For this review, take the finished solid that the model builds, in its own axes (mm). Coordinates: 2 decimals unless noted, no trailing zeros. Loops run counter-clockwise (first coordinate to the right, second up) from the corner with the lowest first, then second, coordinate; pieces in that order, holes last. Notation, with made-up numbers: (-36.75, 33) - (11.25, 33) arc R29 cw to (11.25, 61) - close; hole circle Ø5 at (-18, -22). An arc over 180 degrees is marked (long way). One line per item, written item: value. Start each with the question number.
1. Take a section at B-B, the plane x = 0. State the section outline as (y, z) points.
2. To check wall thickness, follow line 1 (Y direction, x = 11.5, z = 11.75); line 2 (Y direction, x = -8, z = 6); line 3 (X direction, y = 11, z = 26.5). State the ranges of each line that lie inside material, in increasing order. Write a range as from..to.
3. The part is to be moulded in two halves that separate along X. For faces 1 (the face through (-8, 8, 29)), 2 (the face through (-12.838, 4.176, 14.297)), say which applies: released by +X, released by -X, zero draft, split by the parting line, or undercut.
4. Insertion check: pin 1 (2 mm diameter, centred on y = -12, z = 19, fed in from -X); pin 2 (3 mm diameter, centred on y = -10, z = 11, fed in from -X); pin 3 (3 mm diameter, centred on x = -3.5, z = 8, fed in from +Y). Each pin has a flat end and moves straight along its axis. Give the tip position at first contact, or say it passes through.
5. Take a section at A-A, the plane y = 0. State the section outline as (x, z) points, and give its area (3 significant figures).
Autodesk Inventor part; units mm, degrees
ref_plane "YZ Plane" through (0, 0, 0) normal (1, 0, 0) x (0, 1, 0)
ref_plane "XZ Plane" through (0, 0, 0) normal (0, 1, 0) x (-1, 0, 0)
ref_plane "XY Plane" through (0, 0, 0) normal (0, 0, 1) x (1, 0, 0)
sketch "Sketch1" plane through (0, 0, 0) normal (0, 0, 1) x (1, 0, 0)
  arc A0 (-10.8205, 1.9793) -> (-10.8147, -2.0103) centre (0, 0) ccw
  line L0 (-10.8147, -2.0103) -> (-13.2812, -2.8117)
  line L1 (-12.3877, -5.5615) -> (-13.2812, -2.8117)
  line L2 (-13.2812, -2.8117) -> (-12.3877, -5.5615)
  line L3 (-12.3877, -5.5615) -> (-9.9173, -4.7588)
  line L4 (-12.3974, 5.5317) -> (-13.2908, 2.782)
  line L5 (-13.2908, 2.782) -> (-10.8205, 1.9793)
  line L6 (-9.931, 4.7303) -> (-12.3974, 5.5317)
  arc A1 (-7.5905, 7.9614) -> (-9.931, 4.7303) centre (0, 0) ccw
  line L7 (-6.7782, 11.7623) -> (-9.1173, 10.0628)
  line L8 (-9.1173, 10.0628) -> (-7.5905, 7.9614)
  line L9 (-5.2539, 9.6642) -> (-6.7782, 11.7623)
  arc A2 (-1.4613, 10.9025) -> (-5.2539, 9.6642) centre (0, 0) ccw
  line L10 (1.43, 13.5) -> (-1.4613, 13.5)
  line L11 (-1.4613, 13.5) -> (-1.4613, 10.9025)
  line L12 (1.43, 10.9067) -> (1.43, 13.5)
  arc A3 (5.2261, 9.6792) -> (1.43, 10.9067) centre (0, 0) ccw
  line L13 (9.092, 10.0812) -> (6.7529, 11.7806)
  line L14 (6.7529, 11.7806) -> (5.2261, 9.6792)
  line L15 (7.5677, 7.9831) -> (9.092, 10.0812)
  arc A4 (9.9173, 4.7588) -> (7.5677, 7.9831) centre (0, 0) ccw
  line L16 (13.2812, 2.8117) -> (12.3877, 5.5615)
  line L17 (12.3877, 5.5615) -> (9.9173, 4.7588)
  line L18 (10.8147, 2.0103) -> (13.2812, 2.8117)
  arc A5 (10.8205, -1.9793) -> (10.8147, 2.0103) centre (0, 0) ccw
  line L19 (12.3974, -5.5317) -> (13.2908, -2.782)
  line L20 (13.2908, -2.782) -> (10.8205, -1.9793)
  line L21 (9.931, -4.7303) -> (12.3974, -5.5317)
  arc A6 (7.5905, -7.9614) -> (9.931, -4.7303) centre (0, 0) ccw
  line L22 (6.7782, -11.7623) -> (9.1173, -10.0628)
  line L23 (9.1173, -10.0628) -> (7.5905, -7.9614)
  line L24 (5.2539, -9.6642) -> (6.7782, -11.7623)
  arc A7 (1.4613, -10.9025) -> (5.2539, -9.6642) centre (0, 0) ccw
  line L25 (-1.43, -13.5) -> (1.4613, -13.5)
  line L26 (1.4613, -13.5) -> (1.4613, -10.9025)
  line L27 (-1.43, -10.9067) -> (-1.43, -13.5)
  arc A8 (-5.2261, -9.6792) -> (-1.43, -10.9067) centre (0, 0) ccw
  line L28 (-9.092, -10.0812) -> (-6.7529, -11.7806)
  line L29 (-6.7529, -11.7806) -> (-5.2261, -9.6792)
  line L30 (-7.5677, -7.9831) -> (-9.092, -10.0812)
  arc A9 (-9.9173, -4.7588) -> (-7.5677, -7.9831) centre (0, 0) ccw
  circle A10 centre (0, 0) radius 17
  circle A11 centre (0, 0) radius 8.5
  point P0 (-10.8205, 1.9793)
  point P1 (-7.5905, 7.9614)
  point P2 (5.2261, 9.6792)
  point P3 (9.9173, 4.7588)
  point P4 (10.8205, -1.9793)
  point P5 (7.5905, -7.9614)
  point P6 (1.4613, -10.9025)
  point P7 (-5.2261, -9.6792)
  point P8 (-9.9173, -4.7588)
  dimension "d2" = 360
  dimension "d3" = 34
  dimension "d6" = 11
  dimension "d7" = 17
  dimension "d8" = 2.5933
  dimension "d9" = 2.8912
extrude "Extrusion1" add sketch "Sketch1" along normal blind 29 contours A10
properties part number "opona"
Solutions:
1. outline: (-17, 0) - (-13.5, 0) - (-13.5, 29) - (-17, 29) - close; (13.5, 0) - (17, 0) - (17, 29) - (13.5, 29) - close
2. line 1: -12.52..-5.24, -2.2..2.23, 5.27..12.52
2. line 2: -15..-10.87, -8.58..-7.55, 7.55..8.53, 10.87..15
2. line 3: -12.96..-7.83, -6.22..-1.46, 1.43..6.19, 7.83..12.96
3. face 1: zero draft
3. face 2: undercut
4. pin 1: x = -12.96
4. pin 2: x = -14.72
4. pin 3: y = 16.88
5. outline: (-17, 0) - (-11, 0) - (-11, 29) - (-17, 29) - close; (11, 0) - (17, 0) - (17, 29) - (11, 29) - close
5. area: 348 mm2
